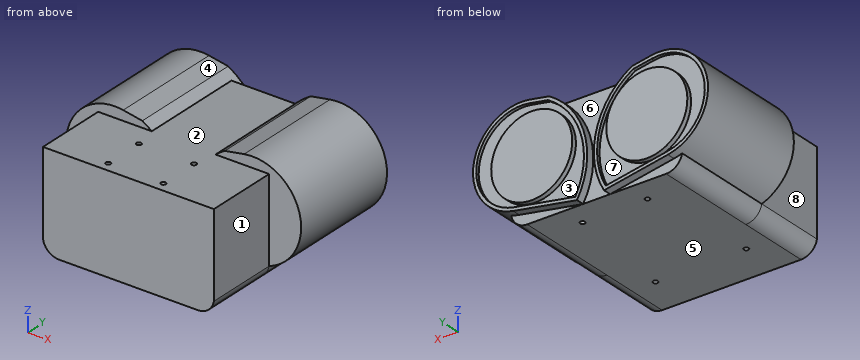
from build123d import *
from build123d.topology import SkipClean

# Parameters (mm, degrees)
SALIENTE_EXTRUIR1_DEPTH        = 60
SALIENTE_EXTRUIR1_DEPTH_BACK   = 10
SALIENTE_EXTRUIR1_2_DEPTH      = 60
SALIENTE_EXTRUIR1_2_DEPTH_BACK = 10
CROQUIS5_W                     = 105.42
CROQUIS5_H                     = 65
SALIENTE_EXTRUIR4_DEPTH        = 60
REDONDEO1_R                    = 10
CORTAR_EXTRUIR3_DEPTH          = 2
CROQUIS8_R                     = 25
SALIENTE_EXTRUIR5_DEPTH        = 3
SALIENTE_EXTRUIR6_DEPTH        = 45
CROQUIS10_R                    = 1.5
CORTAR_EXTRUIR4_DEPTH          = 5
CROQUIS11_R                    = 1.5
CORTAR_EXTRUIR5_DEPTH          = 5


with BuildPart() as part:
    # Croquis1 → Saliente-Extruir1 (new, two sides: drawn at the far end of the back side and taken through both)
    with BuildSketch(Plane(origin=(0, 0, 0), x_dir=(1, 0, 0), z_dir=(0, 1, 0)).offset(-SALIENTE_EXTRUIR1_DEPTH_BACK)):
        with BuildLine():
            Line((-5.20944533, 29.54423259), (34.18286479, 36.490159697))
            ThreePointArc((34.18286479, 36.490159697), (38.849607431, 0.961785341), (17.027138366, -27.460454458))
            Line((17.027138366, -27.460454458), (5.20944533, -29.54423259))
            ThreePointArc((5.20944533, -29.54423259), (-29.54423259, -5.20944533), (-5.20944533, 29.54423259))
        make_face()
    extrude(amount=SALIENTE_EXTRUIR1_DEPTH + SALIENTE_EXTRUIR1_DEPTH_BACK)



with BuildPart() as body_2:
    # Croquis1 → Saliente-Extruir1 2 (new, two sides: drawn at the far end of the back side and taken through both)
    with BuildSketch(Plane(origin=(0, 0, 0), x_dir=(1, 0, 0), z_dir=(0, 1, 0)).offset(-SALIENTE_EXTRUIR1_2_DEPTH_BACK)):
        with BuildLine():
            Line((90.20944533, 29.54423259), (50.81713521, 36.490159697))
            ThreePointArc((50.81713521, 36.490159697), (46.150392569, 0.961785341), (67.972861634, -27.460454458))
            Line((67.972861634, -27.460454458), (79.79055467, -29.54423259))
            ThreePointArc((79.79055467, -29.54423259), (114.54423259, -5.20944533), (90.20944533, 29.54423259))
        make_face()
    extrude(amount=SALIENTE_EXTRUIR1_2_DEPTH + SALIENTE_EXTRUIR1_2_DEPTH_BACK)


with BuildPart() as part_1:
    add(part.part)

    add(body_2.part)  # Saliente-Extruir4 merges body 2
    # Croquis5 → Saliente-Extruir4 (add)
    with BuildSketch(Plane(origin=(0, 0, -36.490159697), x_dir=(-1, 0, 0), z_dir=(0, 0, -1))):
        with Locations((-42.50055467, 22.5)):
            Rectangle(CROQUIS5_W, CROQUIS5_H)
    extrude(amount=-SALIENTE_EXTRUIR4_DEPTH)

    # Redondeo1
    # the kernel refuses this fillet: 10 mm, written as the material it takes off along each edge
    with BuildSketch(Plane(origin=(-10.20944533, 79.627778647, -36.490159697), x_dir=(1, 0, 0), z_dir=(0, -1, 0))) as redondeo1_piece_1:
        with BuildLine():
            CenterArc((9.851111459, 10), REDONDEO1_R, 189.899393553, 80.100606447)
            Line((0, 8.280813266), (-0.197022229, 8.246429532))
            ThreePointArc((-0.197022229, 8.246429532), (-0.2, 4.140406633), (-0.2, 0))
            Line((-0.2, 0), (0, -0.2))
            Line((0, -0.2), (9.851111459, -0.2))
            Line((9.851111459, -0.2), (9.851111459, 0))
        make_face()
    extrude(amount=114.255557294, mode=Mode.SUBTRACT)
    with BuildSketch(Plane(origin=(95.21055467, -34.627953804, -36.490159697), x_dir=(-1, 0, 0), z_dir=(0, 1, 0))) as redondeo1_piece_2:
        with BuildLine():
            CenterArc((9.851181521, 10), REDONDEO1_R, 189.897058287, 80.102941713)
            Line((0, 8.28121478), (-0.19702363, 8.246839076))
            ThreePointArc((-0.19702363, 8.246839076), (-0.2, 4.14060739), (-0.2, 0))
            Line((-0.2, 0), (0, -0.2))
            Line((0, -0.2), (9.851181521, -0.2))
            Line((9.851181521, -0.2), (9.851181521, 0))
        make_face()
    extrude(amount=114.255907607, mode=Mode.SUBTRACT)

    # Croquis7 → Cortar-Extruir3 (cut)
    with BuildSketch(Plane(origin=(0, 60, 0), x_dir=(1, 0, 0), z_dir=(0, 1, 0))):
        with BuildLine():
            Line((4.862148975, -27.574617084), (16.328937751, -25.552712841))
            ThreePointArc((16.328937751, -25.552712841), (36.779644877, 0.976339149), (33.127899287, 34.273287591))
            Line((33.127899287, 34.273287591), (-4.862148975, 27.574617084))
            ThreePointArc((-4.862148975, 27.574617084), (-27.574617084, -4.862148975), (4.862148975, -27.574617084))
        make_face()
        with BuildLine():
            Line((89.862148975, 27.574617084), (51.872100713, 34.273287591))
            ThreePointArc((51.872100713, 34.273287591), (48.220355123, 0.976339149), (68.671062249, -25.552712841))
            Line((68.671062249, -25.552712841), (80.137851025, -27.574617084))
            ThreePointArc((80.137851025, -27.574617084), (112.574617084, -4.862148975), (89.862148975, 27.574617084))
        make_face()
    extrude(amount=-CORTAR_EXTRUIR3_DEPTH, mode=Mode.SUBTRACT)

    # Croquis8 → Saliente-Extruir5 (add)
    with BuildSketch(Plane(origin=(0, 58, 0), x_dir=(1, 0, 0), z_dir=(0, 1, 0))):
        with Locations(Location((7, 3, 0), (0, 0, 270))):
            Circle(CROQUIS8_R)
        with Locations(Location((78, 3, 0), (0, 0, 270))):
            Circle(CROQUIS8_R)
    extrude(amount=SALIENTE_EXTRUIR5_DEPTH)

    # Croquis9 → Saliente-Extruir6 (add)
    with SkipClean():  # the faces are left unmerged after this step: merging them gives an invalid solid
        with BuildSketch(Plane.XZ.offset(10)):
            with BuildLine():
                ThreePointArc((85.359373149, -36.490159697), (91.794128303, -34.144826646), (95.21055467, -28.208944917))
                Line((95.21055467, -28.208944917), (95.21055467, 23.509840303))
                Line((95.21055467, 23.509840303), (62.176934943, 23.509840303))
                Line((62.176934943, 23.509840303), (22.823065057, 23.509840303))
                Line((22.823065057, 23.509840303), (-10.20944533, 23.509840303))
                Line((-10.20944533, 23.509840303), (-10.20944533, -28.209346431))
                ThreePointArc((-10.20944533, -28.209346431), (-6.79293303, -34.144957779), (-0.358333871, -36.490159697))
                Line((-0.358333871, -36.490159697), (85.359373149, -36.490159697))
            make_face()
        extrude(amount=SALIENTE_EXTRUIR6_DEPTH)

    # Croquis10 → Cortar-Extruir4 (cut)
    with SkipClean():  # the faces are left unmerged after this step: merging them gives an invalid solid
        with BuildSketch(Plane.XY.offset(23.509840303)):
            with Locations((59.50055467, -24)):
                Circle(CROQUIS10_R)
            with Locations((59.50055467, -49)):
                Circle(CROQUIS10_R)
            with Locations((25.50055467, -24)):
                Circle(CROQUIS10_R)
            with Locations((25.50055467, -49)):
                Circle(CROQUIS10_R)
        extrude(amount=-CORTAR_EXTRUIR4_DEPTH, mode=Mode.SUBTRACT)

    # Croquis11 → Cortar-Extruir5 (cut)
    with SkipClean():  # the faces are left unmerged after this step: merging them gives an invalid solid
        with BuildSketch(Plane(origin=(0, 0, -36.490159697), x_dir=(-1, 0, 0), z_dir=(0, 0, -1))):
            with Locations((-62.500519639, 40)):
                Circle(CROQUIS11_R)
            with Locations((-22.500519639, 40)):
                Circle(CROQUIS11_R)
            with Locations((-14.500519639, -30)):
                Circle(CROQUIS11_R)
            with Locations((-70.500519639, -30)):
                Circle(CROQUIS11_R)
        extrude(amount=-CORTAR_EXTRUIR5_DEPTH, mode=Mode.SUBTRACT)


solid = part_1.part
Work out the finished part from the listing and answer in its coordinate system (mm). Face numbers are marked on the shaded views. A direction names the side the tool comes from. Give positions to 0.01 mm unless a question says otherwise; leave off trailing zeros. Order: outer loops, then holes, each group sorted by start corner. A loop starts at its lowest first (then second) coordinate and runs counter-clockwise, first axis right, second up. Notation, with made-up numbers: (83, 56.25) -> (110, 56.25) arc R18 cw to (110, 67.25) -> close; hole circle Ø2 at (30, 59.25). An arc over 180 degrees is marked (long way). Answer as a JSON object with one key per item and string values. Group by question number.
1. Section C-C on z = -3 is taken. Determine the outline of the cut face in (x, y), plus the area to 3 significant figures.
2. Section D-D on y = -16.5 is taken. Determine the outline of the cut face in (x, z), plus the area to 3 significant figures.
3. Section B-B on x = 7 is taken. Determine the outline of the cut face in (y, z), plus the area to 3 significant figures.
4. The mould has two halves that part along X. Classify the marked faces 5, 6, 7 and 8: released by +X, released by -X, zero draft, split by the parting line, or undercut.
5. Flat-ended cylindrical pins translate along their axes: pin 1 Ø3 at (x, y) = (97, -27) entering from +Z; pin 2 Ø0.9 at (x, y) = (59, -48.5) entering from +Z; pin 3 Ø4 at (x, z) = (66, -30.5) entering from +Y; pin 4 Ø1 at (y, z) = (-19.5, 10) entering from -X. Find the tip coordinate at first contact, or state that the pin passes through.
6. Section A-A on y = -2.5 is taken. Determine the outline of the cut face in (x, z).
7. Consider line 1 along Y through (x, z) = (55.5, 23); line 2 along Z through (x, y) = (28.5, 6); line 3 along X through (y, z) = (-45.5, 12). Determine where each line is inside the solid, lowest interval first. Write a range as [from, to].
8. A tool of negligible diameter and unlimited length cuts with its end or side. For the marked faces 1, 2, 3 and 4, from which of +Z, -Z, +X, -X, +Y, -Y can it reach the whole face along a straight path? Write none if from no direction.
Result sheet:
{
 "1": {"outline": "(-29.85, -10) -> (-10.21, -10) -> (-10.21, -55) -> (95.21, -55) -> (95.21, -10) -> (114.85, -10) -> (114.85, 60) -> (112.84, 60) -> (112.84, 58) -> (103, 58) -> (103, 61) -> (53, 61) -> (53, 58) -> (47.7, 58) -> (47.7, 60) -> (45.65, 60) -> (45.65, 55) -> (39.35, 55) -> (39.35, 60) -> (37.3, 60) -> (37.3, 58) -> (32, 58) -> (32, 61) -> (-18, 61) -> (-18, 58) -> (-27.84, 58) -> (-27.84, 60) -> (-29.85, 60) -> close", "area": "14,900 mm^2"},
 "2": {"outline": "(-10.21, -28.21) arc R10 ccw to (-0.36, -36.49) -> (85.36, -36.49) arc R10 ccw to (95.21, -28.21) -> (95.21, 23.51) -> (-10.21, 23.51) -> close", "area": "6,280 mm^2"},
 "3": {"outline": "(-55, -36.49) -> (55, -36.49) -> (55, -31.7) -> (60, -31.7) -> (60, -29.67) -> (58, -29.67) -> (58, -28) -> (61, -28) -> (61, 22) -> (58, 22) -> (58, 27.2) -> (60, 27.2) -> (60, 29.23) -> (-10, 29.23) -> (-10, 23.51) -> (-55, 23.51) -> close", "area": "7,310 mm^2"},
 "4": {"face 5": "zero draft", "face 6": "undercut", "face 7": "undercut", "face 8": "released by -X"},
 "5": {"pin 1": "passes through", "pin 2": "stops at z = 18.51", "pin 3": "stops at y = 60", "pin 4": "stops at x = -10.21"},
 "6": {"outline": "(-10.21, -28.21) arc R10 ccw to (-0.36, -36.49) -> (85.36, -36.49) arc R10 ccw to (95.21, -28.21) arc R30 ccw to (79.79, 29.54) -> (67.97, 27.46) arc R46.82 ccw to (62.18, 23.51) -> (22.82, 23.51) arc R46.82 ccw to (17.03, 27.46) -> (5.21, 29.54) arc R30 ccw to start"},
 "7": {"line 1": "y = [-55, 55]", "line 2": "z = [-36.49, 23.51]", "line 3": "x = [-10.21, 95.21]"},
 "8": {"face 1": "+Z, -Z, +X, -Y", "face 2": "+Z, -Y", "face 3": "+Y", "face 4": "+Z, +Y, -Y"}
}
